from build123d import *

# Parameters (mm, degrees)
ESQUISSE1_R             = 20
BOSS_EXTRU_1_DEPTH      = 41
ESQUISSE2_R             = 10
ESQUISSE2_R_2           = 7
BOSS_EXTRU_2_DEPTH      = 5
ESQUISSE3_R             = 3
BOSS_EXTRU_3_DEPTH      = 17
ESQUISSE4_R             = 1.25
ENL_V_MAT_EXTRU_1_DEPTH = 7.9


with BuildPart() as part:
    # Esquisse1 → Boss.-Extru.1 (new body)
    with BuildSketch(Plane.XY):
        Circle(ESQUISSE1_R)
    extrude(amount=-BOSS_EXTRU_1_DEPTH)

    # Esquisse2 → Boss.-Extru.2 (add)
    with BuildSketch(Plane.XY):
        Circle(ESQUISSE2_R)
        Circle(ESQUISSE2_R_2, mode=Mode.SUBTRACT)
    extrude(amount=BOSS_EXTRU_2_DEPTH)

    # Esquisse3 → Boss.-Extru.3 (add)
    with BuildSketch(Plane.XY):
        Circle(ESQUISSE3_R)
    extrude(amount=BOSS_EXTRU_3_DEPTH)

    # Esquisse4 → Enlèv. mat.-Extru.1 (cut)
    with BuildSketch(Plane.XY):
        with Locations((0, 15.05)):
            Circle(ESQUISSE4_R)
        with Locations((13.033682327, -7.525)):
            Circle(ESQUISSE4_R)
        with Locations((-13.033682327, -7.525)):
            Circle(ESQUISSE4_R)
    extrude(amount=-ENL_V_MAT_EXTRU_1_DEPTH, mode=Mode.SUBTRACT)


solid = part.part
Source: CAD feature listing. Evaluate the final solid. Frame: model axes, mm. A direction names the side the tool comes from. Coordinates: 2 decimals unless noted, no trailing zeros. Loops run counter-clockwise (first coordinate to the right, second up) from the corner with the lowest first, then second, coordinate; pieces in that order, holes last. Notation, with made-up numbers: M -35.5,56 L -15.5,56 A19 ccw -15.5,63 Z; hole C -35,41.5 d1. An arc over 180 degrees is marked long. Answer in a Markdown table with one row per item.
Q1. Section A-A on x = 0. Return the cut outline in (y, z).
Answers below:
| item | result |
|---|---|
| outline | M -20,-41 L 20,-41 L 20,0 L 16.3,0 L 16.3,-7.9 L 13.8,-7.9 L 13.8,0 L 10,0 L 10,5 L 7,5 L 7,0 L 3,0 L 3,17 L -3,17 L -3,0 L -7,0 L -7,5 L -10,5 L -10,0 L -20,0 Z |
Q2. Section B-B on y = 0. Return the cut outline in (x, z).
Answers below:
| item | result |
|---|---|
| outline | M -20,-41 L 20,-41 L 20,0 L 10,0 L 10,5 L 7,5 L 7,0 L 3,0 L 3,17 L -3,17 L -3,0 L -7,0 L -7,5 L -10,5 L -10,0 L -20,0 Z |
Q3. Section C-C on z = 7.5. Return the cut outline in (x, y), plus the area to 3 significant figures.
Answers below:
| item | result |
|---|---|
| outline | C 0,0 d6 |
| area | 28.3 mm^2 |
Q4. Ray query, probe 1 along Y at (x, z) = (0, 3); probe 2 along Z at (x, y) = (-13, 1); probe 3 along Y at (x, z) = (14, -33.5). Return the intervals inside material, ascending. Write a range as from..to.
Answers below:
| item | result |
|---|---|
| probe 1 | y = -10..-7, -3..3, 7..10 |
| probe 2 | z = -41..0 |
| probe 3 | y = -14.28..14.28 |
Q5. Draft query along X for faces 3 (the flat face through (-7, -2, 5)), 4 (the cylindrical face through (-4.336, -19.524, -20.213)), 5 (the flat face through (1, -3, 0)). Return one class per face: pulls with the +X half, pulls with the -X half, needs draft (parallel to the pull), parting line crosses it, or undercut.
Answers below:
| item | result |
|---|---|
| face 3 | needs draft |
| face 4 | parting line crosses it |
| face 5 | undercut |
Q6. Set-up query: faces 1 (the flat face through (0, 0, 17)), 2 (the cylindrical face through (6.466, -2.681, 2.465)). Return all of +Z, -Z, +X, -X, +Y, -Y with unobstructed straight access to the full face (end or side cutting, diameter ignored); none if empty.
Answers below:
| item | result |
|---|---|
| face 1 | +Z, +X, -X, +Y, -Y |
| face 2 | +Z |
Q7. First-contact query: pin 1 (1.2 mm diameter, centred on x = 0, y = 14.5, fed in from +Z); pin 2 (3 mm diameter, centred on x = 0, y = 15.05, fed in from +Z); pin 3 (5 mm diameter, centred on x = 9.5, z = -10, fed in from +Y) (3 decimals). Flat tips, straight axial feed; report the tip coordinate or a pass-through.
Answers below:
| item | result |
|---|---|
| pin 1 | stops at z = -7.9 |
| pin 2 | stops at z = 0 |
| pin 3 | stops at y = 18.735 |
Q8. Section D-D on y = -5. Return the cut outline in (x, z).
Answers below:
| item | result |
|---|---|
| outline | M -19.36,-41 L 19.36,-41 L 19.36,0 L 8.66,0 L 8.66,5 L 4.9,5 L 4.9,0 L -4.9,0 L -4.9,5 L -8.66,5 L -8.66,0 L -19.36,0 Z |
